The listing builds one solid part. Answer for the finished solid, in the listing's coordinates (mm). A direction names the side the tool comes from. Give positions to 0.01 mm unless a question says otherwise; leave off trailing zeros. Write each loop counter-clockwise with the first axis right and the second up, starting at its lowest first coordinate (ties: lowest second). Pieces come first, ordered by that corner, then holes. Notation, with made-up numbers: M 82,17.5 L 121,17.5 A11 ccw 121,30.5 Z; hole C 38.25,20 d8. An arc over 180 degrees is marked long. Return JSON: item names as keys, results as strings.
Autodesk Inventor part; units mm, degrees
ref_plane "YZ Plane" through (0, 0, 0) normal (1, 0, 0) x (0, 1, 0)
ref_plane "XZ Plane" through (0, 0, 0) normal (0, 1, 0) x (-1, 0, 0)
ref_plane "XY Plane" through (0, 0, 0) normal (0, 0, 1) x (1, 0, 0)
sketch "Sketch1" plane through (0, 0, 0) normal (0, 0, 1) x (1, 0, 0)
  arc A0 (14.865, 0) -> (-14.865, 0) centre (0, 0) ccw
  arc A1 (17.1039, 3) -> (-17.1039, 3) centre (0, 0) ccw
  line L0 (-17.1039, 3) -> (-29.865, 3)
  line L1 (-29.865, 3) -> (-29.865, 0)
  line L2 (-29.865, 0) -> (-14.865, 0)
  line L3 (14.865, 0) -> (29.865, 0)
  line L4 (29.865, 0) -> (29.865, 3)
  line L5 (29.865, 3) -> (17.1039, 3)
  arc A2 (1.4092, 13.8937) -> (-1.4092, 13.8937) centre (0, 0) ccw
  line L6 (-1.4092, 13.8937) -> (-1.5, 14.7891)
  line L7 (1.4092, 13.8937) -> (1.5, 14.7891)
  point P0 (0, 13.965)
  dimension "d0" = 3
  dimension "d1" = 14.865
  dimension "d3" = 2.5
  dimension "d8" = 15
  dimension "d17" = 0.9
  dimension "d18" = 3
extrude "Extrusion1" add sketch "Sketch1" along normal blind 15
sketch "Sketch2" plane through (-29.865, 0, 0) normal (0, -1, 0) x (1, 0, 0)
  line L0 (0, 15) -> (15, 15)
  line L1 (0, 0) -> (0, 15)
  point P0 (29.865, 0)
  point P1 (7.5, 7.5)
  point P2 (7.5, 15)
  point P3 (0, 7.5)
hole "Hole1" at (-22.365, 0, 7.5) direction (0, 1, 0) diameter 3 end through all
mirror "Mirror1" about plane through (0, 0, 0) normal (1, 0, 0) of "Hole1"
fillet "Fillet1" radius 4 4 edges at (-29.865, 1.5, 0) (-29.865, 1.5, 15) (29.865, 1.5, 15) (29.865, 1.5, 0)
properties part number "Motor Mount C-Clamp Top"
Item 1: A cutting plane is placed at B-B, the plane y = 9.25. Write down the section's boundary in (x, z).
Geometry results:
{"outline": "M -14.7,0 L -11.64,0 L -11.64,15 L -14.7,15 Z; M 11.64,0 L 14.7,0 L 14.7,15 L 11.64,15 Z"}
Item 2: Find the intervals of material crossed by line 1 (X direction, y = 1.85, z = 7.5) (3 decimals); line 2 (X direction, y = 0.7, z = 7.5) (1 decimal); line 3 (Y direction, x = 0.5, z = 10), in increasing order.
Geometry results:
{"line 1": "x = -29.865 to -23.865, -20.865 to -14.749, 14.749 to 20.865, 23.865 to 29.865", "line 2": "x = -29.9 to -23.9, -20.9 to -14.8, 14.8 to 20.9, 23.9 to 29.9", "line 3": "y = 13.96 to 17.36"}
Item 3: Determine the mould class of faces 1 (the cylindrical face through (-21.45, 1.52, 8.69)), 2 (the cylindrical face through (28.72, 1.52, 1.2)), 3 (the cylindrical face through (-28.72, 1.48, 1.2)) for opening direction X: +X half, -X half, draft (parallel to the pull), parting line (faces both ways), or undercut.
Geometry results:
{"face 1": "undercut", "face 2": "+X half", "face 3": "-X half"}
Item 4: Which of the six approach directions +Z, -Z, +X, -X, +Y, -Y give full straight-line access (tool end or side, diameter ignored) to faces 4 (the flat face through (25, 3, 7)), 5 (the cylindrical face through (-11, 10, 7)), 6 (the flat face through (-25, 3, 7))?
Geometry results:
{"face 4": "+Z, -Z, +X, +Y", "face 5": "+Z, -Z, -Y", "face 6": "+Z, -Z, -X, +Y"}
Item 5: A cutting plane is placed at A-A, the plane z = 7.5. Write down the section's boundary in (x, y) (3 decimals), plus the area to 3 significant figures.
Geometry results:
{"outline": "M -29.865,0 L -23.865,0 L -23.865,3 L -29.865,3 Z; M -20.865,0 L -14.865,0 A14.865 cw -1.5,14.789 L -1.409,13.894 A13.965 cw 1.409,13.894 L 1.5,14.789 A14.865 cw 14.865,0 L 20.865,0 L 20.865,3 L 17.104,3 A17.365 ccw -17.104,3 L -20.865,3 Z; M 23.865,0 L 29.865,0 L 29.865,3 L 23.865,3 Z", "area": "187 mm2"}
Item 6: Given pin 1 Ø6 at (y, z) = (11.5, 10) entering from -X; pin 2 Ø2.5 at (x, z) = (22.365, 7.5) entering from +Y; pin 3 Ø4 at (y, z) = (8, 9.5) entering from -X; pin 4 Ø6.5 at (x, z) = (26, 8.5) entering from +Y, each flat-ended and moving along its own axis, determine where each tip first touches the part or whether it passes through.
Geometry results:
{"pin 1": "stops at x = -15.14", "pin 2": "passes through", "pin 3": "stops at x = -16.3", "pin 4": "stops at y = 3"}
Item 7: A cutting plane is placed at C-C, the plane z = 14. Write down the section's boundary in (x, y) (3 decimals), plus the area to 3 significant figures.
Geometry results:
{"outline": "M -28.511,0 L -14.865,0 A14.865 cw -1.5,14.789 L -1.409,13.894 A13.965 cw 1.409,13.894 L 1.5,14.789 A14.865 cw 14.865,0 L 28.511,0 L 28.511,3 L 17.104,3 A17.365 ccw -17.104,3 L -28.511,3 Z", "area": "197 mm2"}
Item 8: A cutting plane is placed at D-D, the plane x = -19. Write down the section's boundary in (y, z), plus the area to 3 significant figures.
Geometry results:
{"outline": "M 0,0 L 3,0 L 3,15 L 0,15 Z", "area": "45.0 mm2"}
